from build123d import *

# Parameters (mm, degrees)
F1_DEPTH       = 5.08
F2_T1_DEPTH    = 62.1438386925
F2_T3_DEPTH    = 62.1438386925
F2_T6_ANGLE    = 166.0840890898
F2_T8_ANGLE    = 196.1575929171
F3_T1_DEPTH    = 62.1438386925
F3_T3_DEPTH    = 62.1438386925
F3_T6_ANGLE    = 166.0840890898
F3_T8_ANGLE    = 196.1575929171
F5_D           = 5
F5_CSINK_D     = 10
F5_CSINK_ANGLE = 90
F6_D           = 4


# Not quite as in the source:
# - a fillet or chamfer that OpenCascade refuses, or shapes differently, is made with other operations: its cross-section is extruded or revolved along the edge and cut away or added


with BuildPart() as f1:
    # F0 (on Front) → F1 (new body)
    with BuildSketch(Plane.XZ):
        with BuildLine():
            Line((57.4674687515, 10.7454937358), (4.2709509748, 17.237583418))
            Line((4.2709509748, 17.237583418), (0, 17.7588092034))
            ThreePointArc((0, 17.7588092034), (-17.7588092034, 0), (0, -17.7588092034))
            Line((0, -17.7588092034), (4.2709509748, -17.237583418))
            Line((4.2709509748, -17.237583418), (57.4674687515, -10.7454937358))
            ThreePointArc((57.4674687515, -10.7454937358), (66.9813094594, 0), (57.4674687515, 10.7454937358))
        make_face()
    extrude(amount=F1_DEPTH)

    # F2: fillet of radius 1 on 4 edges, made by hand

    # F2_s2 → F2_t1 (cut)
    with BuildSketch(Plane(origin=(-6.354175572, 0, 0.7754619925), x_dir=(0, 1, 0), z_dir=(0.992635314, 0, -0.1211409647))):
        with BuildLine():
            ThreePointArc((-5.08, 16.6280211506), (-4.7871067812, 17.3351279318), (-4.08, 17.6280211506))
            Line((-4.08, 17.6280211506), (-5.08, 17.6280211506))
            Line((-5.08, 17.6280211506), (-5.08, 16.6280211506))
        make_face()
    extrude(amount=F2_T1_DEPTH, mode=Mode.SUBTRACT)

    # F2_s4 → F2_t3 (cut)
    with BuildSketch(Plane(origin=(55.3319932641, 0, 6.7527025749), x_dir=(0, 1, 0), z_dir=(-0.992635314, 0, -0.1211409647))):
        with BuildLine():
            ThreePointArc((-5.08, 16.6280211506), (-4.7871067812, 17.3351279318), (-4.08, 17.6280211506))
            Line((-4.08, 17.6280211506), (-5.08, 17.6280211506))
            Line((-5.08, 17.6280211506), (-5.08, 16.6280211506))
        make_face()
    extrude(amount=F2_T3_DEPTH, mode=Mode.SUBTRACT)

    # F2_s5 → F2_t6 (revolve, cut)
    with BuildSketch(Plane(origin=(55.3319932641, 0, 6.7527025749), x_dir=(0, 1, 0), z_dir=(-0.992635314, 0, -0.1211409647))):
        with BuildLine():
            ThreePointArc((-4.08, 17.6280211506), (-4.7871067812, 17.3351279318), (-5.08, 16.6280211506))
            Line((-5.08, 16.6280211506), (-5.08, 17.6280211506))
            Line((-5.08, 17.6280211506), (-4.08, 17.6280211506))
        make_face()
    revolve(axis=Axis((56.156091392, -5.08, 0), (0, -1, 0)), revolution_arc=F2_T6_ANGLE, mode=Mode.SUBTRACT)

    # F2_s7 → F2_t8 (revolve, cut)
    with BuildSketch(Plane(origin=(0, 0, 0), x_dir=(0, 1, 0), z_dir=(0.9900757335, 0, -0.1405348426))):
        with BuildLine():
            ThreePointArc((-5.08, 16.7588092034), (-4.7871067812, 17.4659159846), (-4.08, 17.7588092034))
            Line((-4.08, 17.7588092034), (-5.08, 17.7588092034))
            Line((-5.08, 17.7588092034), (-5.08, 16.7588092034))
        make_face()
    revolve(axis=Axis((0, -5.08, 0), (0, -1, 0)), revolution_arc=F2_T8_ANGLE, mode=Mode.SUBTRACT)

    # F3: fillet of radius 1 on 4 edges, made by hand

    # F3_s2 → F3_t1 (cut)
    with BuildSketch(Plane(origin=(55.3319932641, 0, -6.7527025749), x_dir=(0, 1, 0), z_dir=(-0.992635314, 0, 0.1211409647))):
        with BuildLine():
            ThreePointArc((0, -16.6280211506), (-0.2928932188, -17.3351279318), (-1, -17.6280211506))
            Line((-1, -17.6280211506), (0, -17.6280211506))
            Line((0, -17.6280211506), (0, -16.6280211506))
        make_face()
    extrude(amount=F3_T1_DEPTH, mode=Mode.SUBTRACT)

    # F3_s4 → F3_t3 (cut)
    with BuildSketch(Plane(origin=(-6.354175572, 0, -0.7754619925), x_dir=(0, 1, 0), z_dir=(0.992635314, 0, 0.1211409647))):
        with BuildLine():
            ThreePointArc((0, -16.6280211506), (-0.2928932188, -17.3351279318), (-1, -17.6280211506))
            Line((-1, -17.6280211506), (0, -17.6280211506))
            Line((0, -17.6280211506), (0, -16.6280211506))
        make_face()
    extrude(amount=F3_T3_DEPTH, mode=Mode.SUBTRACT)

    # F3_s5 → F3_t6 (revolve, cut)
    with BuildSketch(Plane(origin=(55.3319932641, 0, 6.7527025749), x_dir=(0, 1, 0), z_dir=(-0.992635314, 0, -0.1211409647))):
        with BuildLine():
            ThreePointArc((-1, 17.6280211506), (-0.2928932188, 17.3351279318), (0, 16.6280211506))
            Line((0, 16.6280211506), (0, 17.6280211506))
            Line((0, 17.6280211506), (-1, 17.6280211506))
        make_face()
    revolve(axis=Axis((56.156091392, 0, 0), (0, -1, 0)), revolution_arc=F3_T6_ANGLE, mode=Mode.SUBTRACT)

    # F3_s7 → F3_t8 (revolve, cut)
    with BuildSketch(Plane(origin=(0, 0, 0), x_dir=(0, 1, 0), z_dir=(0.9900757335, 0, -0.1405348426))):
        with BuildLine():
            ThreePointArc((0, 16.7588092034), (-0.2928932188, 17.4659159846), (-1, 17.7588092034))
            Line((-1, 17.7588092034), (0, 17.7588092034))
            Line((0, 17.7588092034), (0, 16.7588092034))
        make_face()
    revolve(axis=Axis((0, 0, 0), (0, -1, 0)), revolution_arc=F3_T8_ANGLE, mode=Mode.SUBTRACT)

    # F5 (through all)
    with Locations(Plane.XZ.offset(5.08)):
        with Locations((0, 0)):
            CounterSinkHole(F5_D / 2, F5_CSINK_D / 2, counter_sink_angle=F5_CSINK_ANGLE)

    # F6 (through all)
    with Locations(Plane.XZ.offset(5.08)):
        with Locations((56.156091392, 0)):
            Hole(F6_D / 2)


solid = f1.part
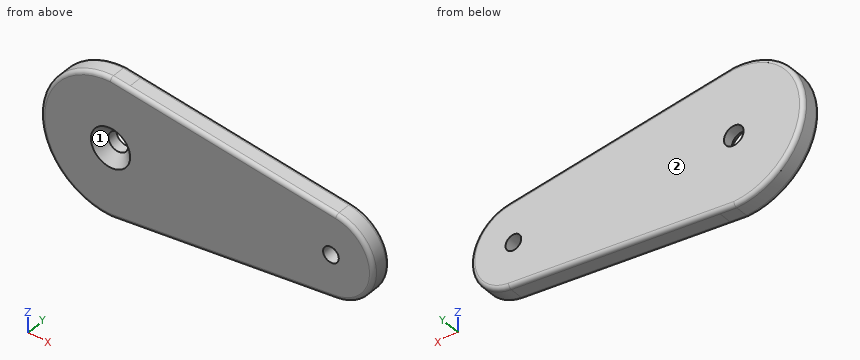
Can you work these out from the model? Positions are in its coordinate system, mm. Face numbers are marked on the shaded views. Give positions to 0.01 mm unless a question says otherwise; leave off trailing zeros. Order: outer loops, then holes, each group sorted by start corner. A loop starts at its lowest first (then second) coordinate and runs counter-clockwise, first axis right, second up. Notation, with made-up numbers: M 22,-23.5 L 35,-23.5 A12 cw 35,-5.5 Z; hole C 62.5,62 d3. An arc over 180 degrees is marked long. Use one line per item in the form item = value.
Item 1: Will these pins go through, and if not, where does the flat tip stop? pin 1 Ø2 at (x, y) = (16, -4) entering from +Z; pin 2 Ø3 at (y, z) = (-2, -9.5) entering from -X; pin 3 Ø5 at (x, z) = (56.16, 0) entering from +Y; pin 4 Ø1.5 at (y, z) = (-3.5, -5.5) entering from +X.
Values follow:
pin_1 = 15.93
pin_2 = -15.85
pin_3 = 0
pin_4 = 65.88
Item 2: Thinking about a two-plate mould opening in Z: for the marked faces 1 and 2, which applies, pulls with the +Z half, pulls with the -Z half, needs draft (parallel to the pull), parting line crosses it, or undercut?
Values follow:
face_1 = undercut
face_2 = needs draft
Item 3: If I drill on line 1 along Z through (x, y) = (0, -1.95); line 2 along Z through (x, y) = (57, -4.8); line 3 along Z through (x, y) = (5, -1.95), over which ranges is the centre line in solid material (lowest first)? Write a range as [from, to].
Values follow:
line_1 = [-17.76, -2.5], [2.5, 17.76]
line_2 = [-10.49, -1.81], [1.81, 10.49]
line_3 = [-17.15, 17.15]
Item 4: If we section it at A-A, the plane z = 0: Write out the boundary of the cut face in (x, y).
Values follow:
outline = M -17.76,-4.08 A1 ccw -16.76,-5.08 L -5,-5.08 L -2.5,-2.58 L -2.5,0 L -16.76,0 A1 ccw -17.76,-1 Z; M 2.5,-2.58 L 5,-5.08 L 54.16,-5.08 L 54.16,0 L 2.5,0 Z; M 58.16,-5.08 L 65.98,-5.08 A1 ccw 66.98,-4.08 L 66.98,-1 A1 ccw 65.98,0 L 58.16,0 Z
